Geometry check sheet. Reference: drawing and pictorial views, mm from the part's lowest x, y, z. A direction names the side the tool comes from. Give positions to 0.01 mm unless a question says otherwise; leave off trailing zeros. Order: outer loops, then holes, each group sorted by start corner. A loop starts at its lowest first (then second) coordinate and runs counter-clockwise, first axis right, second up.
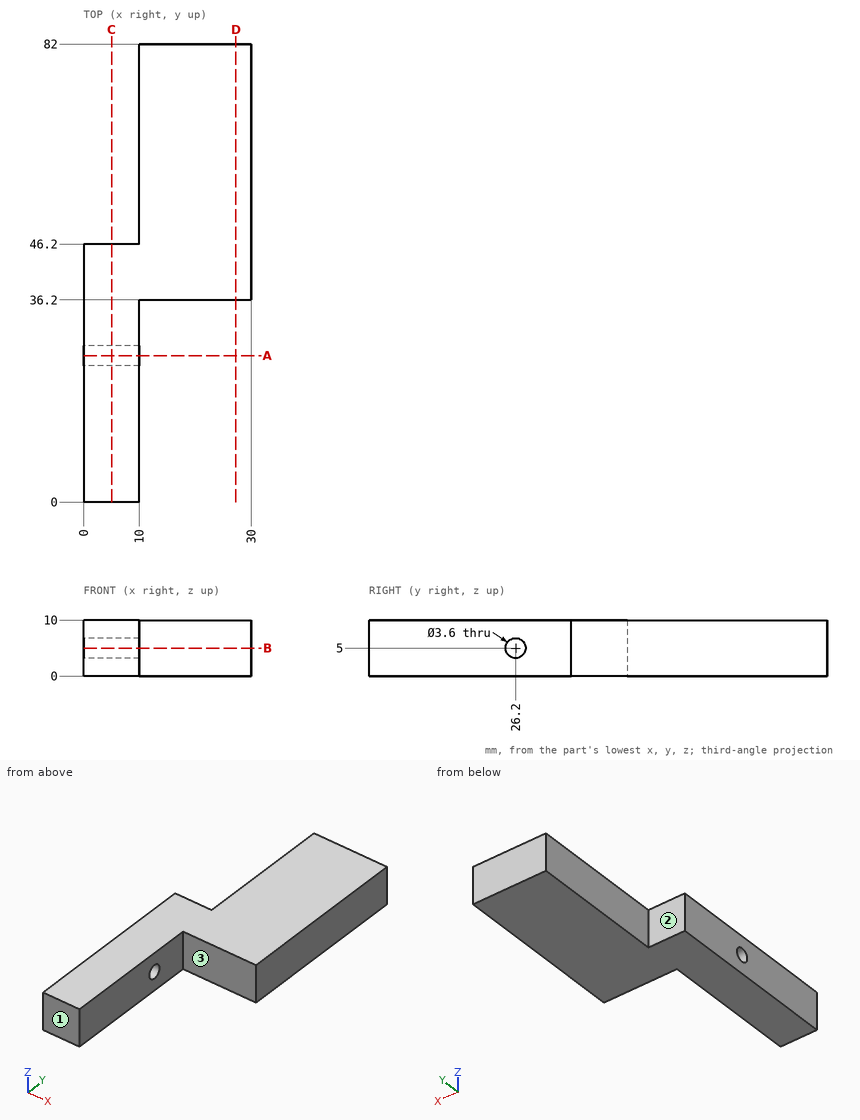
1) Set-up check for the marked faces 1, 2 and 3: record each of +Z, -Z, +X, -X, +Y, -Y from which the full face is reachable in a straight line by a thin tool's end or side.
Recorded:
face 1: +Z, -Z, +X, -X, -Y
face 2: +Z, -Z, -X, +Y
face 3: +Z, -Z, +X, -Y
2) Section check A-A, the plane y = 26.2. Record the cut outline in (x, z).
Recorded:
outline: (0, 0) - (10, 0) - (10, 3.2) - (0, 3.2) - close; (0, 6.8) - (10, 6.8) - (10, 10) - (0, 10) - close
3) Material ranges on L1, parallel to Y at x = 6.5, z = 5; L2, parallel to Z at x = 7.75, y = 26.2; L3, parallel to Y at x = 7.75, z = 1.25, recorded low to high.
Recorded:
L1: y = 0 to 24.4, 28 to 46.2
L2: z = 0 to 3.2, 6.8 to 10
L3: y = 0 to 46.2
4) Depth check by flat-ended pin: pin 1 Ø5 at (y, z) = (61.5, 5) entering from -X; pin 2 Ø5 at (x, z) = (6.5, 5.5) entering from +Y; pin 3 Ø3 at (x, z) = (15, 6.5) entering from -Y. Enter the tip coordinate at first touch or a pass-through.
Recorded:
pin 1: stops at x = 10
pin 2: stops at y = 46.2
pin 3: stops at y = 36.2
5) Section check D-D, the plane x = 27.25. Record the cut outline in (y, z), then the cut area to 3 significant figures.
Recorded:
outline: (36.2, 0) - (82, 0) - (82, 10) - (36.2, 10) - close
area: 458 mm2
6) Section check B-B, the plane z = 5. Record the cut outline in (x, y).
Recorded:
outline: (0, 0) - (10, 0) - (10, 24.4) - (0, 24.4) - close; (0, 28) - (10, 28) - (10, 36.2) - (30, 36.2) - (30, 82) - (10, 82) - (10, 46.2) - (0, 46.2) - close
7) Section check C-C, the plane x = 5. Record the cut outline in (y, z), then the cut area to 3 significant figures.
Recorded:
outline: (0, 0) - (46.2, 0) - (46.2, 10) - (0, 10) - close; hole circle Ø3.6 at (26.2, 5)
area: 452 mm2
